Answer from the drawing. Dimensions are ordinates in mm from the lowest x, y and z of the part. Round coordinates to 2 decimals unless told otherwise and drop trailing zeros. Loops run counter-clockwise (first coordinate to the right, second up) from the corner with the lowest first, then second, coordinate; pieces in that order, holes last. Notation, with made-up numbers: M 69,3 L 127,3 A32 cw 127,33 Z; hole C -5.5,53 d3. An arc over 180 degrees is marked long. Answer as a JSON object with one key per item and string values.
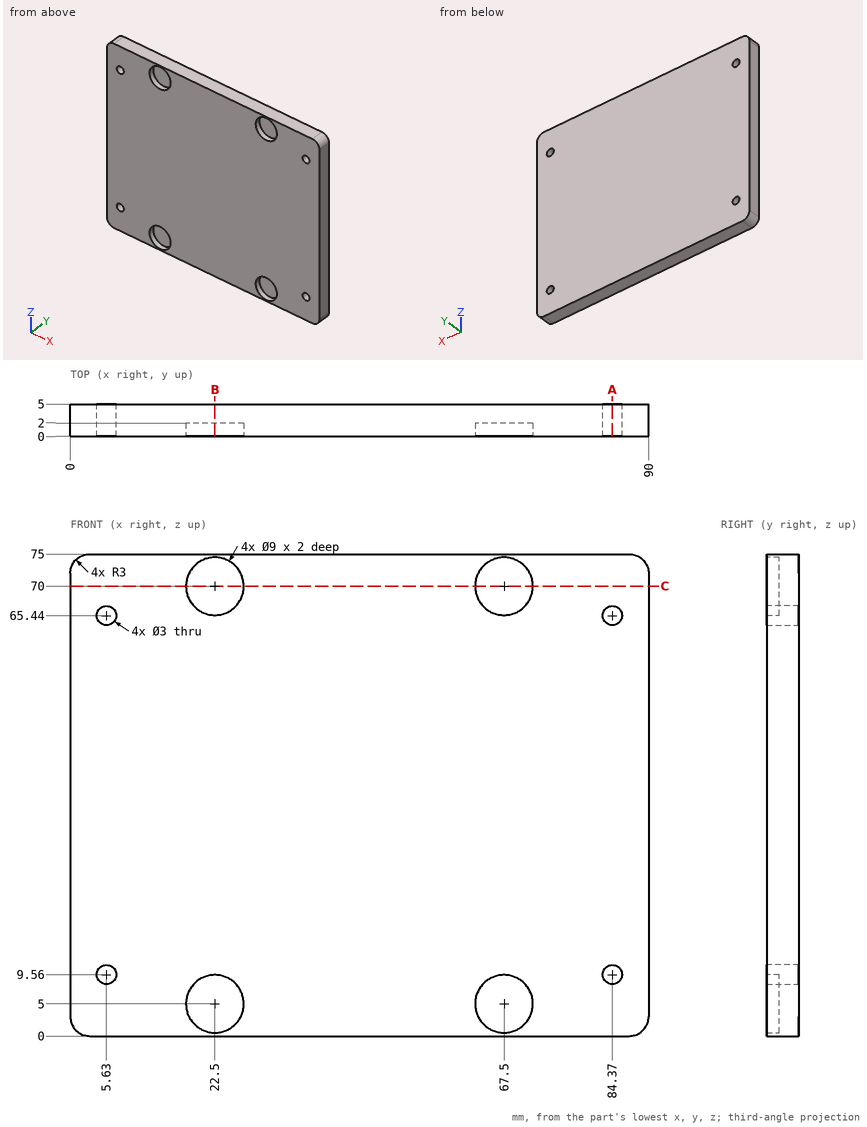
Item 1: Flat-ended cylindrical pins translate along their axes: P1, Ø2.5, axis at x = 66, z = 71, coming from the -Y side; P2, Ø1.8, axis at x = 5.63, z = 65.44, coming from the +Y side. Find the tip coordinate at first contact, or state that the pin passes through.
Values follow:
{"P1": "y = 2", "P2": "through"}
Item 2: The part is cut by section C-C (z = 70). Give the vertices of the cut face in (x, y).
Values follow:
{"outline": "M 0,0 L 18,0 L 18,2 L 27,2 L 27,0 L 63,0 L 63,2 L 72,2 L 72,0 L 90,0 L 90,5 L 0,5 Z"}
Item 3: Straight lines are drawn through the part: line 1 (X direction, y = 2.8, z = 9.56); line 2 (X direction, y = 1.1, z = 5); line 3 (Z direction, x = 21.5, y = 0.6). For each, find the intervals that lie inside material, in ascending order.
Values follow:
{"line 1": "0 to 4.13, 7.13 to 82.87, 85.87 to 90", "line 2": "0 to 18, 27 to 63, 72 to 90", "line 3": "0 to 0.61, 9.39 to 65.61, 74.39 to 75"}
Item 4: The part is cut by section B-B (x = 22.5). Give the vertices of the cut face in (y, z), then the cut area to 3 significant figures.
Values follow:
{"outline": "M 0,0 L 5,0 L 5,75 L 0,75 L 0,74.5 L 2,74.5 L 2,65.5 L 0,65.5 L 0,9.5 L 2,9.5 L 2,0.5 L 0,0.5 Z", "area": "339 mm^2"}
Item 5: The part is cut by section A-A (x = 84.37). Give the vertices of the cut face in (y, z), then the cut area to 3 significant figures.
Values follow:
{"outline": "M 0,0 L 5,0 L 5,8.06 L 0,8.06 Z; M 0,11.06 L 5,11.06 L 5,63.94 L 0,63.94 Z; M 0,66.94 L 5,66.94 L 5,75 L 0,75 Z", "area": "345 mm^2"}
